```python
from build123d import *

# Parameters (mm, degrees)
ESQUISSE1_W                       = 35
ESQUISSE1_H                       = 35
BOSS_EXTRU_1_DEPTH                = 26.5
ESQUISSE2_R                       = 11
BOSS_EXTRU_2_DEPTH                = 2
BOSS_EXTRU_3_DEPTH                = 19
DIAM_TRE_DU_PER_AGE_3_0_3_1_D     = 3
DIAM_TRE_DU_PER_AGE_3_0_3_1_DEPTH = 4.2
DIAM_TRE_DU_PER_AGE_3_0_3_1_TIP   = 0.901290929
CONG_1_R                          = 2.5
ENL_V_START                       = 11
ENL_V_MAT_EXTRU_1_DEPTH           = 5.5
ESQUISSE5_R                       = 0.7
ESQUISSE5_R_2                     = 0.654723083
BOSS_EXTRU_4_DEPTH                = 10


with BuildPart() as part:
    # Esquisse1 → Boss.-Extru.1 (new body)
    with BuildSketch(Plane(origin=(0, 0, 0), x_dir=(1, 0, 0), z_dir=(0, 1, 0))):
        Rectangle(ESQUISSE1_W, ESQUISSE1_H)
    extrude(amount=BOSS_EXTRU_1_DEPTH)

    # Esquisse2 → Boss.-Extru.2 (add)
    with BuildSketch(Plane(origin=(0, 26.5, 0), x_dir=(1, 0, 0), z_dir=(0, 1, 0))):
        with Locations(Location((0, 0, 0), (0, 0, 270))):
            Circle(ESQUISSE2_R)
    extrude(amount=BOSS_EXTRU_2_DEPTH)

    # Esquisse3 → Boss.-Extru.3 (add)
    with BuildSketch(Plane(origin=(0, 28.5, 0), x_dir=(1, 0, 0), z_dir=(0, 1, 0))):
        with BuildLine():
            Line((-1.5, 2), (1.5, 2))
            ThreePointArc((1.5, 2), (0, -2.5), (-1.5, 2))
        make_face()
    extrude(amount=BOSS_EXTRU_3_DEPTH)

    # Diamètre du perçage Ø3.0 (3)1
    with Locations(Plane(origin=(0, 26.5, 0), x_dir=(1, 0, 0), z_dir=(0, 1, 0))):
        with Locations((-13, 13), (13, 13), (13, -13), (-13, -13)):
            Hole(DIAM_TRE_DU_PER_AGE_3_0_3_1_D / 2, depth=DIAM_TRE_DU_PER_AGE_3_0_3_1_DEPTH)
            with Locations((0, 0, -(DIAM_TRE_DU_PER_AGE_3_0_3_1_DEPTH + DIAM_TRE_DU_PER_AGE_3_0_3_1_TIP / 2))):  # 118° drill point
                Cone(0, DIAM_TRE_DU_PER_AGE_3_0_3_1_D / 2, DIAM_TRE_DU_PER_AGE_3_0_3_1_TIP, mode=Mode.SUBTRACT)

    # Congé1
    cong_1_edges = [part.edges().sort_by_distance(p)[0] for p in [
        (-17.5, 13.25, -17.5),
        (17.5, 13.25, -17.5),
        (17.5, 13.25, 17.5),
        (-17.5, 13.25, 17.5),
    ]]
    fillet(cong_1_edges, radius=CONG_1_R)

    # Esquisse4 → Enlèv. mat.-Extru.1 (cut)
    with BuildSketch(Plane(origin=(0, 0, 0), x_dir=(1, 0, 0), z_dir=(0, 1, 0)).offset(ENL_V_START)):
        Polygon((-12.5, 17.5), (-17.5, 12.5), (-17.5, 17.5), align=None)
        Polygon((17.5, 17.5), (12.5, 17.5), (17.5, 12.5), align=None)
        Polygon((12.5, -17.5), (17.5, -12.5), (17.5, -17.5), align=None)
        Polygon((-17.5, -17.5), (-12.5, -17.5), (-17.5, -12.5), align=None)
    extrude(amount=ENL_V_MAT_EXTRU_1_DEPTH, mode=Mode.SUBTRACT)

    # Esquisse5 → Boss.-Extru.4 (add)
    with BuildSketch(Plane.ZY.offset(17.5)):
        with Locations(Location((-1, 7, 0), (0, 0, 180))):
            Circle(ESQUISSE5_R)
        with Locations(Location((-1, 5, 0), (0, 0, 180))):
            Circle(ESQUISSE5_R_2)
        with Locations(Location((1, 5, 0), (0, 0, 180))):
            Circle(ESQUISSE5_R_2)
        with Locations(Location((1, 7, 0), (0, 0, 180))):
            Circle(ESQUISSE5_R)
    extrude(amount=BOSS_EXTRU_4_DEPTH)


solid = part.part
```
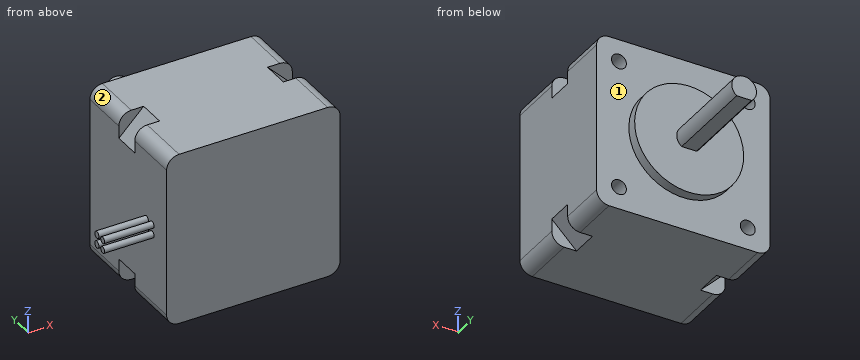
Model file for the job. Use its own axes, mm. Face numbers are marked on the shaded views. A direction names the side the tool comes from. Coordinates: 2 decimals unless noted, no trailing zeros. Order: outer loops, then holes, each group sorted by start corner. A loop starts at its lowest first (then second) coordinate and runs counter-clockwise, first axis right, second up. Notation, with made-up numbers: (26.5, 1.5) - (67.5, 1.5) arc R6 cw to (67.5, 12.5) - close; hole circle Ø6 at (29, 80). An arc over 180 degrees is marked (long way). Return JSON: item names as keys, results as strings. Group by question number.
1) Tool access for the marked faces 1 and 2: list every direction of +Z, -Z, +X, -X, +Y, -Y with a clear straight run to the whole face (end or side of a thin tool).
2) Saw through at D-D, the plane x = 0. Write the cut outline in (y, z), plus the area to 3 significant figures.
3) Probe line 1 (Z direction, x = 13, y = 24.55); line 2 (X direction, y = 21.5, z = -10). List the from-to ranges inside material, lowest first. Write a range as from..to.
4) Flat gauge pins, fed straight in: P1, Ø13, axis at y = 16.5, z = -3.5, coming from the -X side; P2, Ø5.5, axis at x = -14.5, z = -15, coming from the -Y side; P3, Ø4, axis at x = -14.5, z = -15.5, coming from the +Y side; P4, Ø2.5, axis at x = -13, z = 13, coming from the +Y side. Where does each tip first touch, or does it go through?
5) Saw through at A-A, the plane y = 7. Write the cut outline in (x, z), plus the area to 3 significant figures.
6) Saw through at B-B, the plane x = -23. Write the cut outline in (y, z), plus the area to 3 significant figures.
7) Saw through at C-C, the plane z = 1. Write the cut outline in (x, y), plus the area to 3 significant figures.
Values found:
{
 "1": {"face 1": "+Y", "face 2": "+Z, -X, +Y, -Y"},
 "2": {"outline": "(0, -17.5) - (26.5, -17.5) - (26.5, -11) - (28.5, -11) - (28.5, -2) - (47.5, -2) - (47.5, 2.5) - (28.5, 2.5) - (28.5, 11) - (26.5, 11) - (26.5, 17.5) - (0, 17.5) - close", "area": "1,060 mm²"},
 "3": {"line 1": "z = -17.5..-14.5, -11.5..11.5, 14.5..17.5", "line 2": "x = -17.5..17.5"},
 "4": {"P1": "stops at x = -17.5", "P2": "stops at y = 0", "P3": "stops at y = 26.5", "P4": "stops at y = 22.15"},
 "5": {"outline": "(-27.5, -1.7) - (-17.5, -1.7) - (-17.5, -15) arc R2.5 ccw to (-15, -17.5) - (15, -17.5) arc R2.5 ccw to (17.5, -15) - (17.5, 15) arc R2.5 ccw to (15, 17.5) - (-15, 17.5) arc R2.5 ccw to (-17.5, 15) - (-17.5, 1.7) - (-27.5, 1.7) - (-27.5, 0.3) - (-17.5, 0.3) - (-17.5, -0.3) - (-27.5, -0.3) - close", "area": "1,250 mm²"},
 "6": {"outline": "circle Ø1.31 at (5, -1); circle Ø1.31 at (5, 1); circle Ø1.4 at (7, -1); circle Ø1.4 at (7, 1)", "area": "5.77 mm²"},
 "7": {"outline": "(-27.5, 4.35) - (-17.5, 4.35) - (-17.5, 0) - (17.5, 0) - (17.5, 26.5) - (10.95, 26.5) - (10.95, 28.5) - (2.29, 28.5) - (2.29, 47.5) - (-2.29, 47.5) - (-2.29, 28.5) - (-10.95, 28.5) - (-10.95, 26.5) - (-17.5, 26.5) - (-17.5, 7.7) - (-27.5, 7.7) - (-27.5, 6.3) - (-17.5, 6.3) - (-17.5, 5.65) - (-27.5, 5.65) - close", "area": "1,090 mm²"}
}
